Design review of the part built by this model. Coordinates are the model's own, in mm. A direction names the side the tool comes from. Give positions to 0.01 mm unless a question says otherwise; leave off trailing zeros. Write each loop counter-clockwise with the first axis right and the second up, starting at its lowest first coordinate (ties: lowest second). Pieces come first, ordered by that corner, then holes. Notation, with made-up numbers: M 76,-30.5 L 118,-30.5 A30 cw 118,-4.5 Z; hole C -27.5,-33.5 d4. An arc over 180 degrees is marked long. Answer in a Markdown table with one row per item.
```python
from build123d import *

# Parameters (mm, degrees)
BOSS_EXTRUDE1_DEPTH = 26
SHELL1_START        = -10
SHELL1_OUTLINE_W    = 20
SHELL1_OUTLINE_H    = 362
SHELL1_DEPTH        = 20
FILLET1_R           = 3
SKETCH3_R           = 4
CUT_EXTRUDE1_DEPTH  = 3
SKETCH4_R           = 4
CUT_EXTRUDE2_DEPTH  = 37


# Read off the part's stored shape, not the designer's step: Shell1
with BuildPart() as part:
    # Sketch2 → Boss-Extrude1 (new body)
    with BuildSketch(Plane(origin=(0, 0, 0), x_dir=(1, 0, 0), z_dir=(0, 1, 0))):
        Polygon((-13, 181), (-43, 181), (-43, 178), (-13, 178), (-13, -181), (13, -181), (13, 178), (43, 178), (43, 181), (13, 181), align=None)
    extrude(amount=BOSS_EXTRUDE1_DEPTH)

    # Shell1 outline → Shell1 (cut)
    with BuildSketch(Plane.YZ.offset(SHELL1_START)):
        with Locations((13, 0)):
            Rectangle(SHELL1_OUTLINE_W, SHELL1_OUTLINE_H)
    extrude(amount=SHELL1_DEPTH, mode=Mode.SUBTRACT)

    # Fillet1
    fillet1_edges = [part.edges().sort_by_distance(p)[0] for p in [
        (-13, 13, -178),
        (13, 13, -178),
        (10, 13, -181),
        (-10, 13, -181),
    ]]
    fillet(fillet1_edges, radius=FILLET1_R)

    # Sketch3 → Cut-Extrude1 (cut)
    with BuildSketch(Plane.XY.offset(-178)):
        with Locations((29.5, 13)):
            Circle(SKETCH3_R)
        with Locations(Location((-29.5, 13, 0), (0, 0, 180))):
            Circle(SKETCH3_R)
    extrude(amount=-CUT_EXTRUDE1_DEPTH, mode=Mode.SUBTRACT)

    # Sketch4 → Cut-Extrude2 (cut)
    with BuildSketch(Plane(origin=(0, 26, 0), x_dir=(1, 0, 0), z_dir=(0, 1, 0))):
        with Locations(Location((0, -3, 0), (0, 0, 270))):
            Circle(SKETCH4_R)
    extrude(amount=-CUT_EXTRUDE2_DEPTH, mode=Mode.SUBTRACT)


solid = part.part
```
1) For faces 1 (the face through (-13, 13, 1)), 2 (the face through (0, 23, -3)), 3 (the face through (26, 10, -178)), 4 (the face through (-1.532, 24.521, 6.695)), list the 3-axis set-ups (+Z, -Z, +X, -X, +Y, -Y) from which the entire face can be reached by the end or side of a thin tool; tool diameter is ignored.
Geometry says:
| item | result |
|---|---|
| face 1 | +Z, -X, +Y, -Y |
| face 2 | +Z, -Z |
| face 3 | +Z, +X, +Y, -Y |
| face 4 | +Y, -Y |
2) To check wall thickness, follow probe 1 along X at (y, z) = (21, -122); probe 2 along X at (y, z) = (23.85, 3); probe 3 along Y at (x, z) = (-29.5, -179.25). State the ranges of each line that lie inside material, in increasing order. Write a range as [from, to].
Geometry says:
| item | result |
|---|---|
| probe 1 | [-13, -10], [10, 13] |
| probe 2 | [-13, -4], [4, 13] |
| probe 3 | [0, 9], [17, 26] |
3) Add section C-C (y = 13). Write out the cut boundary in (x, z), and give its area (3 significant figures).
Geometry says:
| item | result |
|---|---|
| outline | M -43,-181 L -33.5,-181 L -33.5,-178 L -43,-178 Z; M -25.5,-181 L -13,-181 A3 ccw -10,-178 L -10,181 L -13,181 L -13,-175 A3 cw -16,-178 L -25.5,-178 Z; M 10,-178 A3 ccw 13,-181 L 25.5,-181 L 25.5,-178 L 16,-178 A3 cw 13,-175 L 13,181 L 10,181 Z; M 33.5,-181 L 43,-181 L 43,-178 L 33.5,-178 Z |
| area | 2,300 mm^2 |
4) The part is to be moulded in two halves that separate along X. For faces 5 (the face through (1, 1, -181)), 6 (the face through (13, 13, 5)), 7 (the face through (-10, 13, 4)), say which applies: released by +X, released by -X, zero draft, split by the parting line, or undercut.
Geometry says:
| item | result |
|---|---|
| face 5 | zero draft |
| face 6 | released by +X |
| face 7 | undercut |
5) Add section A-A (z = 3). Write out the cut boundary in (x, y).
Geometry says:
| item | result |
|---|---|
| outline | M -13,0 L -4,0 L -4,3 L -10,3 L -10,23 L -4,23 L -4,26 L -13,26 Z; M 4,0 L 13,0 L 13,26 L 4,26 L 4,23 L 10,23 L 10,3 L 4,3 Z |
6) Insertion check: P1, Ø9, axis at x = -29.5, y = 13, coming from the +Z side; P2, Ø12, axis at y = 9.5, z = -86.5, coming from the +X side; P3, Ø12, axis at y = 21.5, z = 25.5, coming from the -X side. Each pin has a flat end and moves straight along its axis. Give the tip position at first contact, or say it passes through.
Geometry says:
| item | result |
|---|---|
| P1 | z = -178 |
| P2 | x = 13 |
| P3 | x = -13 |
7) Add section D-D (x = -29.5). Write out the cut boundary in (y, z).
Geometry says:
| item | result |
|---|---|
| outline | M 0,-181 L 9,-181 L 9,-178 L 0,-178 Z; M 17,-181 L 26,-181 L 26,-178 L 17,-178 Z |
8) Add section B-B (x = 0). Write out the cut boundary in (y, z).
Geometry says:
| item | result |
|---|---|
| outline | M 0,-181 L 3,-181 L 3,-1 L 0,-1 Z; M 0,7 L 3,7 L 3,181 L 0,181 Z; M 23,-181 L 26,-181 L 26,-1 L 23,-1 Z; M 23,7 L 26,7 L 26,181 L 23,181 Z |
